Build history of the part. All positions in model axes, mm. A direction names the side the tool comes from. Round coordinates to 2 decimals unless told otherwise and drop trailing zeros. Write each loop counter-clockwise with the first axis right and the second up, starting at its lowest first coordinate (ties: lowest second). Pieces come first, ordered by that corner, then holes. Notation, with made-up numbers: (60.25, 52) -> (91.25, 52) arc R36 cw to (91.25, 89) -> close; hole circle Ø4 at (27, 28). An arc over 180 degrees is marked (long way). Return JSON: item names as keys, results as strings.
from build123d import *

# Parameters (mm, degrees)
CROQUIS1_W                = 60
CROQUIS1_H                = 160.023288417
SALIENTE_EXTRUIR1_DEPTH   = 7.9375
CROQUIS2_W                = 8.086078182
CROQUIS2_H                = 420
SALIENTE_EXTRUIR2_DEPTH   = 110
CORTAR_EXTRUIR1_DEPTH     = 10
CROQUIS4_W                = 184.389639933
CROQUIS4_H                = 520.028204804
CORTAR_EXTRUIR2_DEPTH     = 10
CONVERTIR_S_LIDO1_START   = -210
CONVERTIR_S_LIDO1_DEPTH   = 420
CONVERTIR_S_LIDO1_2_DEPTH = 420
CORTAR_EXTRUIR3_START     = -117.9375
CORTAR_EXTRUIR3_OUTLINE_W = 14.086078182
CORTAR_EXTRUIR3_OUTLINE_H = 420
CORTAR_EXTRUIR3_DEPTH     = 110
CORTAR_EXTRUIR3_START_2   = -7.9375
CORTAR_EXTRUIR3_2_DEPTH   = 7.9375
CORTAR_EXTRUIR3_3_DEPTH   = 7.9375


# Read off the part's stored shape, not the designer's step: Convertir-Sólido1, Cortar-Extruir3
with BuildPart() as part:
    # Croquis1 → Saliente-Extruir1 (new body)
    # profile 1 of 2: a face of its own
    with BuildSketch(Plane(origin=(0, 0, 0), x_dir=(1, 0, 0), z_dir=(0, 1, 0))):
        Polygon((75, 210), (-75, 210), (-75, 49.976711583), (-75, -210), (75, -210), align=None)
        with BuildLine():
            Line((-57.399097033, -162.050045053), (-57.399097033, -64.544827159))
            Line((-57.399097033, -64.544827159), (-57.399097033, -32.050045053))
            ThreePointArc((-57.399097033, -32.050045053), (-50.012947046, -24.663895066), (-42.626797059, -32.050045053))
            Line((-42.626797059, -32.050045053), (-42.626797059, -64.544827159))
            Line((-42.626797059, -64.544827159), (-42.626797059, -162.050045053))
            Line((-42.626797059, -162.050045053), (-42.626797059, -194.544827159))
            ThreePointArc((-42.626797059, -194.544827159), (-50.012947046, -201.930977146), (-57.399097033, -194.544827159))
            Line((-57.399097033, -194.544827159), (-57.399097033, -162.050045053))
        make_face(mode=Mode.SUBTRACT)
        with BuildLine():
            ThreePointArc((57.373202941, -194.544827159), (49.987052954, -201.930977146), (42.600902967, -194.544827159))
            Line((42.600902967, -194.544827159), (42.600902967, -162.050045053))
            ThreePointArc((42.600902967, -162.050045053), (49.987052954, -154.663895066), (57.373202941, -162.050045053))
            Line((57.373202941, -162.050045053), (57.373202941, -194.544827159))
        make_face(mode=Mode.SUBTRACT)
        with BuildLine():
            ThreePointArc((57.373202941, -64.544827159), (49.987052954, -71.930977146), (42.600902967, -64.544827159))
            Line((42.600902967, -64.544827159), (42.600902967, -32.050045053))
            ThreePointArc((42.600902967, -32.050045053), (49.987052954, -24.663895066), (57.373202941, -32.050045053))
            Line((57.373202941, -32.050045053), (57.373202941, -64.544827159))
        make_face(mode=Mode.SUBTRACT)
        with BuildLine():
            ThreePointArc((-66.642728039, 194.133584854), (-61.642728039, 199.133584854), (-56.642728039, 194.133584854))
            Line((-56.642728039, 194.133584854), (-56.642728039, 74.133584854))
            ThreePointArc((-56.642728039, 74.133584854), (-61.642728039, 69.133584854), (-66.642728039, 74.133584854))
            Line((-66.642728039, 74.133584854), (-66.642728039, 194.133584854))
        make_face(mode=Mode.SUBTRACT)
    # profile 2 of 2: a face of its own
    with BuildSketch(Plane(origin=(0, 0, 0), x_dir=(1, 0, 0), z_dir=(0, 1, 0))):
        with Locations((-105, 129.988355791)):
            Rectangle(CROQUIS1_W, CROQUIS1_H)
        with BuildLine():
            ThreePointArc((-123.366972213, 194.743931483), (-118.366972213, 199.743931483), (-113.366972213, 194.743931483))
            Line((-113.366972213, 194.743931483), (-113.366972213, 74.743931483))
            ThreePointArc((-113.366972213, 74.743931483), (-118.366972213, 69.743931483), (-123.366972213, 74.743931483))
            Line((-123.366972213, 74.743931483), (-123.366972213, 194.743931483))
        make_face(mode=Mode.SUBTRACT)
    extrude(amount=SALIENTE_EXTRUIR1_DEPTH)

    # Croquis2 → Saliente-Extruir2 (add)
    with BuildSketch(Plane.XZ):
        with Locations((4.043039091, 0)):
            Rectangle(CROQUIS2_W, CROQUIS2_H)
    extrude(amount=SALIENTE_EXTRUIR2_DEPTH)

    # Croquis3 → Cortar-Extruir1 (cut)
    with BuildSketch(Plane.ZY):
        with BuildLine():
            Line((-185.90944112, -54.927638628), (-185.90944112, -94.927638628))
            ThreePointArc((-185.90944112, -94.927638628), (-192.40944112, -101.427638628), (-198.90944112, -94.927638628))
            Line((-198.90944112, -94.927638628), (-198.90944112, -54.927638628))
            ThreePointArc((-198.90944112, -54.927638628), (-192.40944112, -48.427638628), (-185.90944112, -54.927638628))
        make_face()
        with BuildLine():
            Line((-125.90944112, -54.927638628), (-125.90944112, -94.927638628))
            ThreePointArc((-125.90944112, -94.927638628), (-132.40944112, -101.427638628), (-138.90944112, -94.927638628))
            Line((-138.90944112, -94.927638628), (-138.90944112, -54.927638628))
            ThreePointArc((-138.90944112, -54.927638628), (-132.40944112, -48.427638628), (-125.90944112, -54.927638628))
        make_face()
        with BuildLine():
            Line((-65.90944112, -54.927638628), (-65.90944112, -94.927638628))
            ThreePointArc((-65.90944112, -94.927638628), (-72.40944112, -101.427638628), (-78.90944112, -94.927638628))
            Line((-78.90944112, -94.927638628), (-78.90944112, -54.927638628))
            ThreePointArc((-78.90944112, -54.927638628), (-72.40944112, -48.427638628), (-65.90944112, -54.927638628))
        make_face()
        with BuildLine():
            Line((-5.90944112, -54.927638628), (-5.90944112, -94.927638628))
            ThreePointArc((-5.90944112, -94.927638628), (-12.40944112, -101.427638628), (-18.90944112, -94.927638628))
            Line((-18.90944112, -94.927638628), (-18.90944112, -54.927638628))
            ThreePointArc((-18.90944112, -54.927638628), (-12.40944112, -48.427638628), (-5.90944112, -54.927638628))
        make_face()
        with BuildLine():
            Line((54.09055888, -54.927638628), (54.09055888, -94.927638628))
            ThreePointArc((54.09055888, -94.927638628), (47.59055888, -101.427638628), (41.09055888, -94.927638628))
            Line((41.09055888, -94.927638628), (41.09055888, -54.927638628))
            ThreePointArc((41.09055888, -54.927638628), (47.59055888, -48.427638628), (54.09055888, -54.927638628))
        make_face()
        with BuildLine():
            Line((114.09055888, -54.927638628), (114.09055888, -94.927638628))
            ThreePointArc((114.09055888, -94.927638628), (107.59055888, -101.427638628), (101.09055888, -94.927638628))
            Line((101.09055888, -94.927638628), (101.09055888, -54.927638628))
            ThreePointArc((101.09055888, -54.927638628), (107.59055888, -48.427638628), (114.09055888, -54.927638628))
        make_face()
        with BuildLine():
            Line((174.09055888, -54.927638628), (174.09055888, -94.927638628))
            ThreePointArc((174.09055888, -94.927638628), (167.59055888, -101.427638628), (161.09055888, -94.927638628))
            Line((161.09055888, -94.927638628), (161.09055888, -54.927638628))
            ThreePointArc((161.09055888, -54.927638628), (167.59055888, -48.427638628), (174.09055888, -54.927638628))
        make_face()
    extrude(amount=-CORTAR_EXTRUIR1_DEPTH, mode=Mode.SUBTRACT)

    # Croquis4 → Cortar-Extruir2 (cut)
    with BuildSketch(Plane.XZ):
        with Locations((100.280898149, 50.014102402)):
            Rectangle(CROQUIS4_W, CROQUIS4_H)
    extrude(amount=-CORTAR_EXTRUIR2_DEPTH, mode=Mode.SUBTRACT)

    # Convertir-Sólido1 outline → Convertir-Sólido1 (cut)
    with BuildSketch(Plane.XY.offset(CONVERTIR_S_LIDO1_START)):
        with BuildLine():
            Line((8.086078182, 7.9375), (-4.851421818, 7.9375))
            ThreePointArc((-4.851421818, 7.9375), (4.296772164, 4.148193982), (8.086078182, -5))
            Line((8.086078182, -5), (8.086078182, 7.9375))
        make_face()
        with BuildLine():
            Line((0, -110), (0.148578182, -110))
            Line((0.148578182, -110), (0.148578182, -5))
            ThreePointArc((0.148578182, -5), (0.11129463, -4.390536748), (0, -3.790162679))
            Line((0, -3.790162679), (0, -110))
        make_face()
    extrude(amount=CONVERTIR_S_LIDO1_DEPTH, mode=Mode.SUBTRACT)

    # Convertir-S_lido1 2 outline → Convertir-S_lido1 2 (add)
    with BuildSketch(Plane.XY.offset(CONVERTIR_S_LIDO1_START)):
        with BuildLine():
            ThreePointArc((-4.851421818, 0), (-1.773206962, -1.059873948), (0, -3.790162679))
            Line((0, -3.790162679), (0, 0))
            Line((0, 0), (-4.851421818, 0))
        make_face()
    extrude(amount=CONVERTIR_S_LIDO1_2_DEPTH)

    # Cortar-Extruir3 outline → Cortar-Extruir3 (cut)
    with BuildSketch(Plane(origin=(0, 7.9375, 0), x_dir=(1, 0, 0), z_dir=(0, 1, 0)).offset(CORTAR_EXTRUIR3_START)):
        with Locations((1.043039091, 0)):
            Rectangle(CORTAR_EXTRUIR3_OUTLINE_W, CORTAR_EXTRUIR3_OUTLINE_H)
    extrude(amount=CORTAR_EXTRUIR3_DEPTH, mode=Mode.SUBTRACT)

    # Cortar-Extruir3 2 outline → Cortar-Extruir3 2 (cut)
    with BuildSketch(Plane(origin=(0, 7.9375, 0), x_dir=(1, 0, 0), z_dir=(0, 1, 0)).offset(CORTAR_EXTRUIR3_START_2)):
        with BuildLine():
            Line((5.19261796, 210), (-0.80738204, 210))
            ThreePointArc((-0.80738204, 210), (2.19261796, 207), (5.19261796, 210))
        make_face()
        with BuildLine():
            Line((-0.80738204, -210), (5.19261796, -210))
            ThreePointArc((5.19261796, -210), (2.19261796, -207), (-0.80738204, -210))
        make_face()
    extrude(amount=CORTAR_EXTRUIR3_2_DEPTH, mode=Mode.SUBTRACT)

    # Cortar-Extruir3 3 outline → Cortar-Extruir3 3 (add)
    with BuildSketch(Plane(origin=(0, 7.9375, 0), x_dir=(1, 0, 0), z_dir=(0, 1, 0)).offset(CORTAR_EXTRUIR3_START_2)):
        with BuildLine():
            ThreePointArc((5.19261796, 210), (2.19261796, 207), (-0.80738204, 210))
            Line((-0.80738204, 210), (-6, 210))
            Line((-6, 210), (-6, -210))
            Line((-6, -210), (-0.80738204, -210))
            ThreePointArc((-0.80738204, -210), (2.19261796, -207), (5.19261796, -210))
            Line((5.19261796, -210), (114.236657738, -210))
            Line((114.236657738, -210), (114.236657738, 210))
            Line((114.236657738, 210), (5.19261796, 210))
        make_face()
        with BuildLine():
            Line((59.164296366, 198.90944112), (99.164296366, 198.90944112))
            ThreePointArc((99.164296366, 198.90944112), (105.664296366, 192.40944112), (99.164296366, 185.90944112))
            Line((99.164296366, 185.90944112), (59.164296366, 185.90944112))
            ThreePointArc((59.164296366, 185.90944112), (52.664296366, 192.40944112), (59.164296366, 198.90944112))
        make_face(mode=Mode.SUBTRACT)
        with BuildLine():
            Line((59.164296366, 138.90944112), (99.164296366, 138.90944112))
            ThreePointArc((99.164296366, 138.90944112), (105.664296366, 132.40944112), (99.164296366, 125.90944112))
            Line((99.164296366, 125.90944112), (59.164296366, 125.90944112))
            ThreePointArc((59.164296366, 125.90944112), (52.664296366, 132.40944112), (59.164296366, 138.90944112))
        make_face(mode=Mode.SUBTRACT)
        with BuildLine():
            Line((59.164296366, 78.90944112), (99.164296366, 78.90944112))
            ThreePointArc((99.164296366, 78.90944112), (105.664296366, 72.40944112), (99.164296366, 65.90944112))
            Line((99.164296366, 65.90944112), (59.164296366, 65.90944112))
            ThreePointArc((59.164296366, 65.90944112), (52.664296366, 72.40944112), (59.164296366, 78.90944112))
        make_face(mode=Mode.SUBTRACT)
        with BuildLine():
            Line((59.164296366, 18.90944112), (99.164296366, 18.90944112))
            ThreePointArc((99.164296366, 18.90944112), (105.664296366, 12.40944112), (99.164296366, 5.90944112))
            Line((99.164296366, 5.90944112), (59.164296366, 5.90944112))
            ThreePointArc((59.164296366, 5.90944112), (52.664296366, 12.40944112), (59.164296366, 18.90944112))
        make_face(mode=Mode.SUBTRACT)
        with BuildLine():
            Line((59.164296366, -41.09055888), (99.164296366, -41.09055888))
            ThreePointArc((99.164296366, -41.09055888), (105.664296366, -47.59055888), (99.164296366, -54.09055888))
            Line((99.164296366, -54.09055888), (59.164296366, -54.09055888))
            ThreePointArc((59.164296366, -54.09055888), (52.664296366, -47.59055888), (59.164296366, -41.09055888))
        make_face(mode=Mode.SUBTRACT)
        with BuildLine():
            Line((59.164296366, -101.09055888), (99.164296366, -101.09055888))
            ThreePointArc((99.164296366, -101.09055888), (105.664296366, -107.59055888), (99.164296366, -114.09055888))
            Line((99.164296366, -114.09055888), (59.164296366, -114.09055888))
            ThreePointArc((59.164296366, -114.09055888), (52.664296366, -107.59055888), (59.164296366, -101.09055888))
        make_face(mode=Mode.SUBTRACT)
        with BuildLine():
            Line((59.164296366, -161.09055888), (99.164296366, -161.09055888))
            ThreePointArc((99.164296366, -161.09055888), (105.664296366, -167.59055888), (99.164296366, -174.09055888))
            Line((99.164296366, -174.09055888), (59.164296366, -174.09055888))
            ThreePointArc((59.164296366, -174.09055888), (52.664296366, -167.59055888), (59.164296366, -161.09055888))
        make_face(mode=Mode.SUBTRACT)
    extrude(amount=CORTAR_EXTRUIR3_3_DEPTH)


solid = part.part
Q1. 3-axis set-ups, long thin cutter, end or side, ignore diameter. For faces 4 (the cylindrical face through (105.663, 3.913, 107.448)), 5 (the flat face through (-105, 4, -49.977)), 6 (the flat face through (16, 0, -3)): which of +Z, -Z, +X, -X, +Y, -Y reach the whole face in a straight line?
Verdict:
{"face 4": "+Y, -Y", "face 5": "+Z, -X, +Y, -Y", "face 6": "+Z, -Z, +X, -X, -Y"}
Q2. Saw through at B-B on x = -50. List the corners of the cut face in (y, z).
Verdict:
{"outline": "(0, -210) -> (7.94, -210) -> (7.94, 24.66) -> (0, 24.66) -> close; (0, 201.93) -> (7.94, 201.93) -> (7.94, 210) -> (0, 210) -> close"}
Q3. Pin check, flat tips, straight feed: pin 1 Ø1.5 at (y, z) = (6.5, -32) entering from -X; pin 2 Ø2 at (x, z) = (-55.5, 134.5) entering from +Y. Stop position of each tip, or through.
Verdict:
{"pin 1": "stops at x = -75", "pin 2": "passes through"}
Q4. Saw through at D-D on y = 4.5. Count the separate pieces of the cut face and the enclosed holes in it, then the cut area to 3 significant figures.
Verdict:
{"separate pieces": "1", "enclosed holes": "10", "area": "79,400 mm²"}
Q5. Saw through at C-C on z = -131.5. List the corners of the cut face in (x, y).
Verdict:
{"outline": "(-135, 0) -> (-123.37, 0) -> (-123.37, 7.94) -> (-135, 7.94) -> close; (-113.37, 0) -> (-66.64, 0) -> (-66.64, 7.94) -> (-113.37, 7.94) -> close; (-56.64, 0) -> (52.73, 0) -> (52.73, 7.94) -> (-56.64, 7.94) -> close; (105.6, 0) -> (114.24, 0) -> (114.24, 7.94) -> (105.6, 7.94) -> close"}
Q6. Two-plate mould, pull along X, no slides. Class faces 1 (the cylindrical face through (52.666, 3.913, 167.733)), 2 (the flat face through (-38, 4, 210)), 3 (the flat face through (114.237, 4, 3)): +X half, -X half, draft (parallel to the pull), parting line (faces both ways), or undercut.
Verdict:
{"face 1": "undercut", "face 2": "draft", "face 3": "+X half"}
Q7. Wall check: L1, parallel to X at y = 2.25, z = -86.5; L2, parallel to X at y = 6.5, z = 127; L3, parallel to X at y = 1.5, z = -77.5. Give the ranges that are in metal, low to high.
Verdict:
{"L1": "x = -135 to -123.37, -113.37 to -66.64, -56.64 to 114.24", "L2": "x = -75 to -57.4, -42.63 to 114.24", "L3": "x = -135 to -123.37, -113.37 to -66.64, -56.64 to 55.12, 103.21 to 114.24"}
Q8. Saw through at A-A on z = 119. List the corners of the cut face in (x, y).
Verdict:
{"outline": "(-75, 0) -> (-57.4, 0) -> (-57.4, 7.94) -> (-75, 7.94) -> close; (-42.63, 0) -> (114.24, 0) -> (114.24, 7.94) -> (-42.63, 7.94) -> close"}
